Here's how the part is built. I have some questions about the finished solid (model axes, mm). Face numbers are marked on the shaded views. A direction names the side the tool comes from. Round coordinates to 2 decimals unless told otherwise and drop trailing zeros. Order: outer loops, then holes, each group sorted by start corner. A loop starts at its lowest first (then second) coordinate and runs counter-clockwise, first axis right, second up. Notation, with made-up numbers: (67.5, -18) -> (83.5, -18) arc R35 ccw to (83.5, 20) -> close; hole circle Ø8 at (76, 57). An arc over 180 degrees is marked (long way). Answer in a Markdown table with one row per item.
Autodesk Inventor part; units mm, degrees
ref_plane "YZ Plane" through (0, 0, 0) normal (1, 0, 0) x (0, 1, 0)
ref_plane "XZ Plane" through (0, 0, 0) normal (0, 1, 0) x (-1, 0, 0)
ref_plane "XY Plane" through (0, 0, 0) normal (0, 0, 1) x (1, 0, 0)
sketch "Sketch1" plane through (0, 0, 0) normal (0, 0, 1) x (1, 0, 0)
  circle A0 centre (0, 0) radius 10
  circle A1 centre (0, 0) radius 17.5
  dimension "d0" = 35
  dimension "d1" = 20
extrude "Extrusion1" add sketch "Sketch1" along normal blind 1
sketch "Sketch2" plane through (0, 0, 1) normal (0, 0, 1) x (1, 0, 0)
  circle A0 centre (-12.1244, 7) radius 1.6
  circle A1 centre (0, 0) radius 10
  circle A2 centre (0, 0) radius 17.5
  line L0 (0, 0) -> (-10, 0) construction
  line L1 (-15.1554, 8.75) -> (-8.6603, 5) construction
  circle A3 centre (0, 0) radius 14 construction
  point P0 (-11.9078, 6.875)
  dimension "d16" = 28
  dimension "d4" = 3.2
  dimension "d8" = 30
extrude "Extrusion2" cut sketch "Sketch2" against normal through all contours A0
sketch "Sketch3" plane through (0, 0, 1) normal (0, 0, 1) x (1, 0, 0)
  circle A0 centre (0, 0) radius 9
  circle A1 centre (0, 0) radius 10
  circle A2 centre (0, 0) radius 10
  dimension "d10" = 1
  dimension "d11" = 20
extrude "Extrusion3" add sketch "Sketch3" along normal blind 8
sketch "Sketch4" plane through (0, 0, 1) normal (0, 0, -1) x (-1, 0, 0)
  circle A0 centre (0, 0) radius 9
  circle A1 centre (0, 0) radius 10
extrude "Extrusion4" add sketch "Sketch4" along normal up to surface (1 mm away)
fillet "Fillet1" radius 1 1 edges at (9, 0, 0)
properties part number "Pre-Anode" material "Stainless Steel"
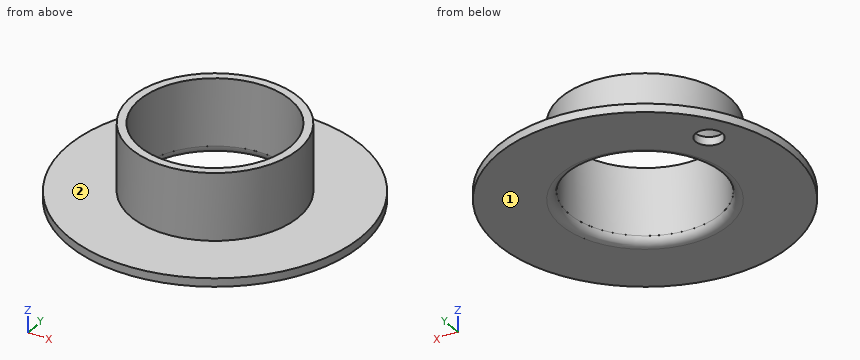
1. Suppose I cut it at C-C on z = 5.5. Write out the boundary of the cut face in (x, y).
Numbers:
| item | result |
|---|---|
| outline | circle Ø20 at (0, 0); hole circle Ø18 at (0, 0) |
2. Please list where these lines run through material, in increasing order: line 1 along Y through (x, z) = (0, 1.05); line 2 along Z through (x, y) = (-14, -1.5); line 3 along Y through (x, z) = (6, 5.5).
Numbers:
| item | result |
|---|---|
| line 1 | y = -10 to -9, 9 to 10 |
| line 2 | z = 0 to 1 |
| line 3 | y = -8 to -6.71, 6.71 to 8 |
3. Suppose I cut it at A-A on y = 0. Write out the boundary of the cut face in (x, z).
Numbers:
| item | result |
|---|---|
| outline | (-17.5, 0) -> (-10, 0) arc R1 ccw to (-9, 1) -> (-9, 9) -> (-10, 9) -> (-10, 1) -> (-17.5, 1) -> close; (9, 1) arc R1 ccw to (10, 0) -> (17.5, 0) -> (17.5, 1) -> (10, 1) -> (10, 9) -> (9, 9) -> close |
4. Suppose I cut it at D-D on x = 14. Write out the boundary of the cut face in (y, z).
Numbers:
| item | result |
|---|---|
| outline | (-10.5, 0) -> (10.5, 0) -> (10.5, 1) -> (-10.5, 1) -> close |
5. For the marked faces 1 and 2, which set-ups out of +Z, -Z, +X, -X, +Y, -Y let a thin tool reach every point of the face, with its end or its side?
Numbers:
| item | result |
|---|---|
| face 1 | -Z, +X, -X, +Y, -Y |
| face 2 | +Z |
6. For pin 1 Ø1.5 at (x, y) = (-14, -7.5) entering from +Z; pin 2 Ø5 at (x, z) = (5, 4.5) entering from +Y; pin 3 Ø2 at (x, y) = (13.5, 5.5) entering from -Z; pin 4 Ø1 at (y, z) = (3.5, 4) entering from +X, each with a flat end and sliding along its axis, tell me the tip position at first contact or that it passes through.
Numbers:
| item | result |
|---|---|
| pin 1 | stops at z = 1 |
| pin 2 | stops at y = 9.68 |
| pin 3 | stops at z = 0 |
| pin 4 | stops at x = 9.54 |
